The figure shows three views and two pictorial views of one solid part (mm, origin at its lowest corner). Answer the questions. A direction names the side the tool comes from. Give positions to 0.01 mm unless a question says otherwise; leave off trailing zeros. Order: outer loops, then holes, each group sorted by start corner. A loop starts at its lowest first (then second) coordinate and runs counter-clockwise, first axis right, second up. Notation, with made-up numbers: (67.5, -9) - (76.5, -9) arc R11 ccw to (76.5, 10) - close; hole circle Ø7 at (-31, 44). An arc over 180 degrees is marked (long way). Write item = value, one per line.
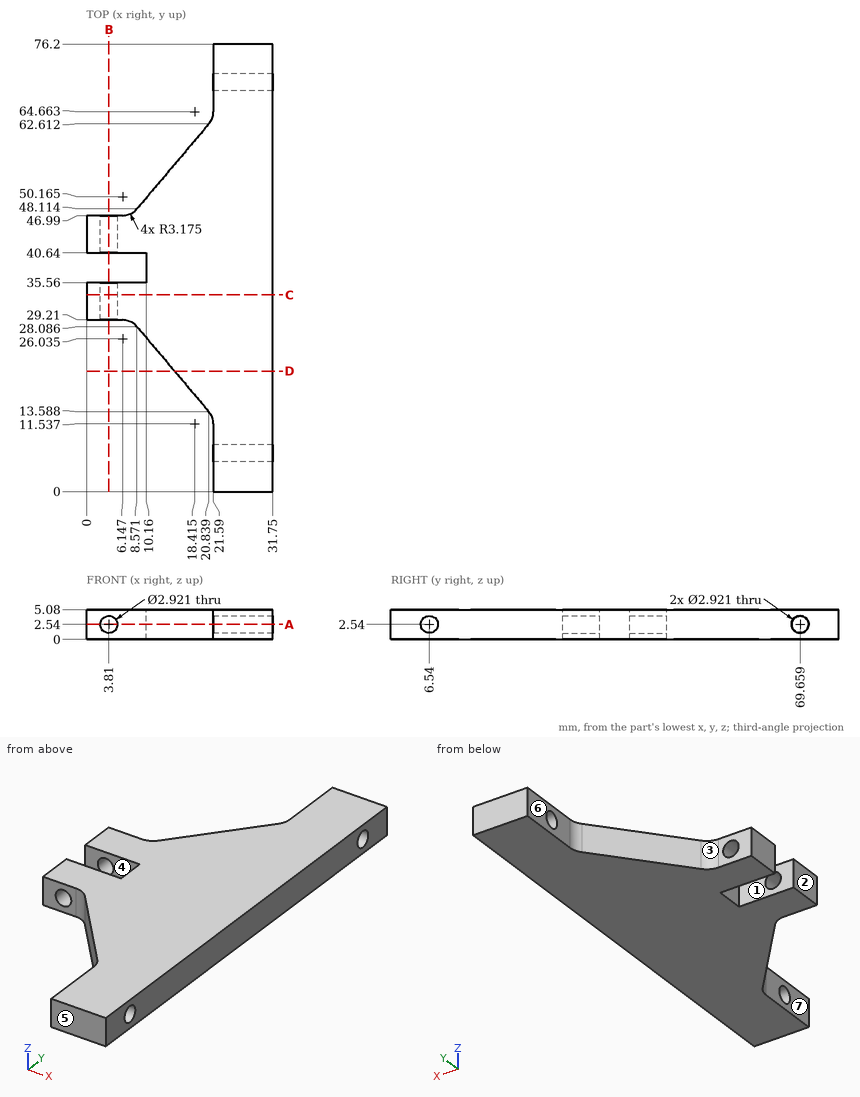
1. For the marked faces 5, 6 and 7, determine the directions among +Z, -Z, +X, -X, +Y, -Y from which every point of the face is accessible in a straight line to the end or side of a thin tool.
Recorded:
face_5 = +Z, -Z, +X, -X, -Y
face_6 = +Z, -Z, -X, +Y
face_7 = +Z, -Z, -X, -Y
2. Section C-C (y = 33.5) is taken. Determine the outline of the cut face in (x, z), and give its area (3 significant figures).
Recorded:
outline = (0, 0) - (31.75, 0) - (31.75, 5.08) - (0, 5.08) - close; hole circle Ø2.92 at (3.81, 2.54)
area = 155 mm^2
3. Section B-B (x = 3.81) is taken. Determine the outline of the cut face in (y, z).
Recorded:
outline = (29.21, 0) - (35.56, 0) - (35.56, 1.08) - (29.21, 1.08) - close; (29.21, 4) - (35.56, 4) - (35.56, 5.08) - (29.21, 5.08) - close; (40.64, 0) - (46.99, 0) - (46.99, 1.08) - (40.64, 1.08) - close; (40.64, 4) - (46.99, 4) - (46.99, 5.08) - (40.64, 5.08) - close
4. Determine the mould class of the marked faces 1, 2, 3 and 4 for opening direction Y: +Y half, -Y half, draft (parallel to the pull), parting line (faces both ways), or undercut.
Recorded:
face_1 = undercut
face_2 = draft
face_3 = +Y half
face_4 = undercut
5. Flat-ended cylindrical pins translate along their axes: pin 1 (1.5 mm diameter, centred on x = 6.5, z = 4, fed in from +Y); pin 2 (1 mm diameter, centred on x = 10, z = 2, fed in from -Y) (1 decimal); pin 3 (1 mm diameter, centred on x = 3, z = 4, fed in from -Y). Find the tip coordinate at first contact, or state that the pin passes through.
Recorded:
pin_1 = 47.19
pin_2 = 25.8
pin_3 = 29.21
6. Straight lines are drawn through the part: L1, parallel to Y at x = 24, z = 2.4 (1 decimal); L2, parallel to Y at x = 24, z = 3.15 (1 decimal); L3, parallel to X at y = 31.25, z = 2.54. For each, find the intervals that lie inside material, in ascending order. Write a range as [from, to].
Recorded:
L1 = [0, 5.1], [8, 68.2], [71.1, 76.2]
L2 = [0, 5.2], [7.9, 68.3], [71, 76.2]
L3 = [0, 2.35], [5.27, 31.75]
7. Section D-D (y = 20.5) is taken. Determine the outline of the cut face in (x, z).
Recorded:
outline = (14.99, 0) - (31.75, 0) - (31.75, 5.08) - (14.99, 5.08) - close
8. Section A-A (z = 2.54) is taken. Count the separate pieces of the cut face and the enclosed holes in it, and give its area (3 significant figures).
Recorded:
separate_pieces = 5
enclosed_holes = 0
area = 1,240 mm^2
